Source: three-view drawing plus pictorial views. Frame: mm from the lowest corner of the part. A direction names the side the tool comes from. Give positions to 0.01 mm unless a question says otherwise; leave off trailing zeros. Loops run counter-clockwise (first coordinate to the right, second up) from the corner with the lowest first, then second, coordinate; pieces in that order, holes last. Notation, with made-up numbers: M 55,-38 L 109,-38 A6 ccw 109,-28 Z; hole C -37,18 d11. An arc over 180 degrees is marked long. Answer as a JSON object with one key per item and string values. Group by question number.
1) Ray query, L1, parallel to X at y = 5, z = 1.15; L2, parallel to Z at x = 10.5, y = 7.25; L3, parallel to Z at x = 5, y = 6. Return the intervals inside material, ascending.
2) Section query D-D on z = 3.5. Return loops of the section in (x, y).
3) Section query A-A on x = 8. Return loops of the section in (y, z), plus the area to 3 significant figures.
4) First-contact query: P1, Ø2, axis at x = 11, y = 5.5, coming from the +Z side; P2, Ø4, axis at y = 8, z = 1, coming from the -X side; P3, Ø4, axis at x = 8, y = 5, coming from the +Z side. Flat tips, straight axial feed; report the tip coordinate or a pass-through.
5) Section query C-C on y = 3.25. Return loops of the section in (x, z) (1 decimal).
6) Draft query along Y for the marked faces 1, 2, 3 and 4. Return one class per face: +Y half, -Y half, draft (parallel to the pull), parting line (faces both ways), or undercut.
7) Section query B-B on z = 1. Count the separate pieces of the cut face and the enclosed holes in it, plus the area to 3 significant figures.
8) Access query for the marked faces 5, 6 and 7. Directions: +Z, -Z, +X, -X, +Y, -Y. A direction counts if a zero-diameter tool reaches every point of the face in a straight line with its end or side. Return the directions, or none.
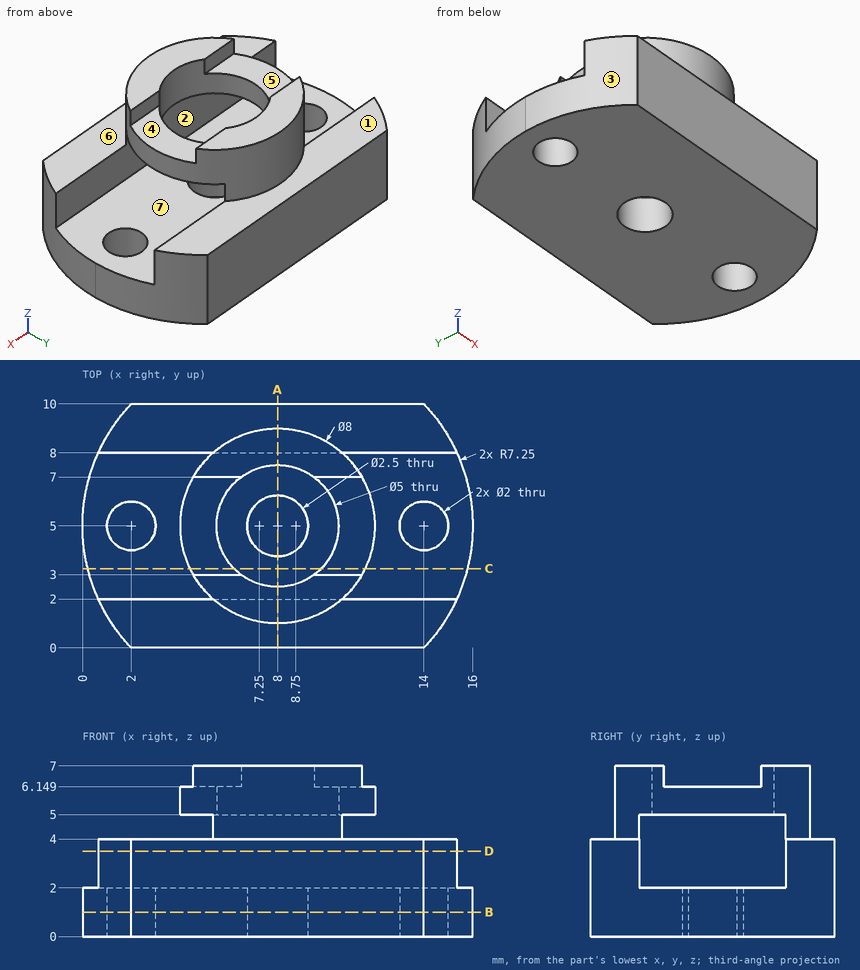
Output:
{
 "1": {"L1": "x = 0 to 1, 3 to 6.75, 9.25 to 13, 15 to 16", "L2": "z = 0 to 2, 5 to 7", "L3": "z = 0 to 2, 5 to 6.15"},
 "2": {"outline": "M 0.65,2 A7.25 ccw 2,0 L 14,0 A7.25 ccw 15.35,2 Z; M 0.65,8 L 15.35,8 A7.25 ccw 14,10 L 2,10 A7.25 ccw Z"},
 "3": {"outline": "M 0,0 L 3.75,0 L 3.75,2 L 2,2 L 2,5 L 2.5,5 L 2.5,7 L 1,7 L 1,4 L 0,4 Z; M 6.25,0 L 10,0 L 10,4 L 9,4 L 9,7 L 7.5,7 L 7.5,5 L 8,5 L 8,2 L 6.25,2 Z", "area": "31.0 mm^2"},
 "4": {"P1": "stops at z = 6.15", "P2": "stops at x = 0.07", "P3": "stops at z = 2"},
 "5": {"outline": "M 0.2,0 L 15.8,0 L 15.8,2 L 0.2,2 Z; M 4.4,5 L 6.2,5 L 6.2,6.1 L 4.4,6.1 Z; M 9.8,5 L 11.6,5 L 11.6,6.1 L 9.8,6.1 Z"},
 "6": {"face 1": "draft", "face 2": "undercut", "face 3": "-Y half", "face 4": "undercut"},
 "7": {"separate pieces": "1", "enclosed holes": "3", "area": "136 mm^2"},
 "8": {"face 5": "+Z, +X, -X", "face 6": "+Z, -Y", "face 7": "+X, -X"}
}
